Design review of the part built by this model. Coordinates are the model's own, in mm. Face numbers are marked on the shaded views. A direction names the side the tool comes from. Coordinates: 2 decimals unless noted, no trailing zeros. Write each loop counter-clockwise with the first axis right and the second up, starting at its lowest first coordinate (ties: lowest second). Pieces come first, ordered by that corner, then holes. Notation, with made-up numbers: (83.5, -23.75) -> (89.5, -23.75) arc R19 ccw to (89.5, -17.75) -> close; hole circle Ø2 at (55, 79.25). An arc over 180 degrees is marked (long way). Return JSON: item names as keys, results as strings. Group by question number.
from build123d import *

# Parameters (mm, degrees)
SALIENTE_EXTRUIR1_DEPTH      = 30
CORTAR_EXTRUIR1_DEPTH        = 5
CROQUIS3_W                   = 30
CROQUIS3_H                   = 25
CORTAR_EXTRUIR2_DEPTH        = 2
CROQUIS4_R                   = 1.35
CROQUIS4_R_2                 = 2.5
CORTAR_EXTRUIR3_DEPTH        = 5
CROQUIS5_W                   = 25
CROQUIS5_H                   = 25
CORTAR_EXTRUIR4_DEPTH        = 2
REDONDEO2_R                  = 20
REDONDEO3_R                  = 8
REDONDEO4_R                  = 2
SALIENTE_EXTRUIR2_DEPTH      = 9
SALIENTE_EXTRUIR2_DEPTH_BACK = 1
CORTAR_EXTRUIR5_START        = 9
CROQUIS10_W                  = 26
CROQUIS10_H                  = 14.6
CORTAR_EXTRUIR5_DEPTH        = 5
SALIENTE_EXTRUIR3_START      = 4
CROQUIS12_R                  = 3.6
CROQUIS12_R_2                = 2.1
SALIENTE_EXTRUIR3_DEPTH      = 3
CORTAR_EXTRUIR7_START        = -2
CROQUIS13_R                  = 2.1
CORTAR_EXTRUIR7_DEPTH        = 5
CORTAR_EXTRUIR8_START        = 9
CROQUIS14_W                  = 26
CROQUIS14_H                  = 5.4
CORTAR_EXTRUIR8_DEPTH        = 3.5
REDONDEO5_R                  = 3
SALIENTE_EXTRUIR4_DEPTH      = 1.5
SALIENTE_EXTRUIR4_DEPTH_BACK = 1.5
SALIENTE_EXTRUIR4_START      = -15


with BuildPart() as part:
    # Croquis1 → Saliente-Extruir1 (new body)
    with BuildSketch(Plane.XY):
        with BuildLine():
            Line((7, 0), (7, 5))
            Line((7, 5), (-33, 5))
            ThreePointArc((-33, 5), (-56.296113, -10.563595), (-70, -35))
            Line((-70, -35), (-70, -80))
            Line((-70, -80), (-65, -80))
            Line((-65, -80), (-65, -34.805195))
            ThreePointArc((-65, -34.805195), (-52.819114, -13.779819), (-32.805195, 0))
            Line((-32.805195, 0), (7, 0))
        make_face()
    extrude(amount=SALIENTE_EXTRUIR1_DEPTH)

    # Croquis2 → Cortar-Extruir1 (cut)
    with BuildSketch(Plane(origin=(0, 5, 0), x_dir=(1, 0, 0), z_dir=(0, 1, 0))):
        with BuildLine():
            Line((-11.4, -6.58), (-1.4, -6.58))
            ThreePointArc((-1.4, -6.58), (-0.05, -7.93), (-1.4, -9.28))
            Line((-1.4, -9.28), (-21.400001, -9.28))
            ThreePointArc((-21.400001, -9.28), (-22.75, -7.93), (-21.4, -6.58))
            Line((-21.4, -6.58), (-11.4, -6.58))
        make_face()
        with BuildLine():
            Line((-1.4, -20.72), (-21.400001, -20.72))
            ThreePointArc((-21.400001, -20.72), (-22.75, -22.07), (-21.4, -23.42))
            Line((-21.4, -23.42), (-11.4, -23.42))
            Line((-11.4, -23.42), (-1.4, -23.42))
            ThreePointArc((-1.4, -23.42), (-0.05, -22.07), (-1.4, -20.72))
        make_face()
    extrude(amount=-CORTAR_EXTRUIR1_DEPTH, mode=Mode.SUBTRACT)

    # Croquis3 → Cortar-Extruir2 (cut)
    with BuildSketch(Plane.XZ):
        with Locations((-11.4, 15)):
            Rectangle(CROQUIS3_W, CROQUIS3_H)
    extrude(amount=-CORTAR_EXTRUIR2_DEPTH, mode=Mode.SUBTRACT)

    # Croquis4 → Cortar-Extruir3 (cut)
    with BuildSketch(Plane.ZY.offset(70)):
        with Locations((22.071068, -54.528932)):
            Circle(CROQUIS4_R)
        with Locations((22.071068, -68.671068)):
            Circle(CROQUIS4_R)
        with Locations((7.928932, -68.671068)):
            Circle(CROQUIS4_R)
        with Locations((7.928932, -54.528932)):
            Circle(CROQUIS4_R)
        with Locations((15, -61.6)):
            Circle(CROQUIS4_R_2)
    extrude(amount=-CORTAR_EXTRUIR3_DEPTH, mode=Mode.SUBTRACT)

    # Croquis5 → Cortar-Extruir4 (cut)
    with BuildSketch(Plane.ZY.offset(70)):
        with Locations((15, -61.6)):
            Rectangle(CROQUIS5_W, CROQUIS5_H)
    extrude(amount=-CORTAR_EXTRUIR4_DEPTH, mode=Mode.SUBTRACT)

    # Redondeo2
    redondeo2_edges = [part.edges().sort_by_distance(p)[0] for p in [
        (-32.805195, 0, 15),
        (-65, -34.805195, 15),
        (-70, -35, 15),
        (-33, 5, 15),
    ]]
    fillet(redondeo2_edges, radius=REDONDEO2_R)

    # Redondeo3
    redondeo3_edges = [part.edges().sort_by_distance(p)[0] for p in [
        (7, 2.5, 0),
        (7, 2.5, 30),
    ]]
    fillet(redondeo3_edges, radius=REDONDEO3_R)

    # Redondeo4
    redondeo4_edges = [part.edges().sort_by_distance(p)[0] for p in [
        (-69, -49.1, 27.5),
        (-69, -74.1, 27.5),
        (-69, -74.1, 2.5),
        (-69, -49.1, 2.5),
        (3.6, 1, 27.5),
        (3.6, 1, 2.5),
        (-26.4, 1, 2.5),
        (-26.4, 1, 27.5),
    ]]
    fillet(redondeo4_edges, radius=REDONDEO4_R)

    # Croquis8 → Saliente-Extruir2 (add, two sides: drawn at the far end of the back side and taken through both)
    with BuildSketch(Plane.ZY.offset(70).offset(-SALIENTE_EXTRUIR2_DEPTH_BACK)):
        with BuildLine():
            Line((2.5, -72.1), (0, -72.1))
            Line((0, -72.1), (0, -80))
            Line((0, -80), (30, -80))
            Line((30, -80), (30, -72.1))
            Line((30, -72.1), (27.5, -72.1))
            ThreePointArc((27.5, -72.1), (26.914214, -73.514214), (25.5, -74.1))
            Line((25.5, -74.1), (4.5, -74.1))
            ThreePointArc((4.5, -74.1), (3.085786, -73.514214), (2.5, -72.1))
        make_face()
        with BuildLine():
            Line((2.5, -51.1), (0, -51.1))
            Line((0, -51.1), (0, -34))
            Line((0, -34), (30, -34))
            Line((30, -34), (30, -51.1))
            Line((30, -51.1), (27.5, -51.1))
            ThreePointArc((27.5, -51.1), (26.914214, -49.685786), (25.5, -49.1))
            Line((25.5, -49.1), (4.5, -49.1))
            ThreePointArc((4.5, -49.1), (3.085786, -49.685786), (2.5, -51.1))
        make_face()
    extrude(amount=SALIENTE_EXTRUIR2_DEPTH + SALIENTE_EXTRUIR2_DEPTH_BACK)

    # Croquis10 → Cortar-Extruir5 (cut)
    with BuildSketch(Plane.ZY.offset(70).offset(CORTAR_EXTRUIR5_START)):
        with Locations((15, -43.8)):
            Rectangle(CROQUIS10_W, CROQUIS10_H)
    extrude(amount=-CORTAR_EXTRUIR5_DEPTH, mode=Mode.SUBTRACT)

    # Croquis12 → Saliente-Extruir3 (add)
    with BuildSketch(Plane.ZY.offset(70).offset(SALIENTE_EXTRUIR3_START)):
        with Locations((5.5, -45.5)):
            Circle(CROQUIS12_R)
        with Locations(Location((5.5, -45.5, 0), (0, 0, 180))):
            Circle(CROQUIS12_R_2, mode=Mode.SUBTRACT)
    extrude(amount=SALIENTE_EXTRUIR3_DEPTH)

    # Croquis13 → Cortar-Extruir7 (cut)
    with BuildSketch(Plane.ZY.offset(74).offset(CORTAR_EXTRUIR7_START)):
        with Locations(Location((5.5, -45.5, 0), (0, 0, 180))):
            Circle(CROQUIS13_R)
    extrude(amount=CORTAR_EXTRUIR7_DEPTH, mode=Mode.SUBTRACT)

    # Croquis14 → Cortar-Extruir8 (cut)
    with BuildSketch(Plane.ZY.offset(70).offset(CORTAR_EXTRUIR8_START)):
        with Locations((15, -74.8)):
            Rectangle(CROQUIS14_W, CROQUIS14_H)
    extrude(amount=-CORTAR_EXTRUIR8_DEPTH, mode=Mode.SUBTRACT)

    # Redondeo5
    redondeo5_edges = [part.edges().sort_by_distance(p)[0] for p in [
        (-72, -80, 30),
        (-74.291633, -34, 30),
        (-74.291633, -34, 0),
        (-72, -80, 0),
    ]]
    fillet(redondeo5_edges, radius=REDONDEO5_R)

    # Croquis15 → Saliente-Extruir4 (add, two sides: drawn at the far end of the back side and taken through both)
    with BuildSketch(Plane.XY.offset(30).offset(SALIENTE_EXTRUIR4_START - SALIENTE_EXTRUIR4_DEPTH_BACK)):
        with BuildLine():
            Line((-65, -38.217888), (-28.4904, 0))
            ThreePointArc((-28.4904, 0), (-33.236938, -0.571403), (-37.712257, -2.252962))
            ThreePointArc((-37.712257, -2.252962), (-53.200641, -14.196528), (-63.566437, -30.782337))
            ThreePointArc((-63.566437, -30.782337), (-64.638339, -34.431646), (-65, -38.217888))
        make_face()
    extrude(amount=SALIENTE_EXTRUIR4_DEPTH + SALIENTE_EXTRUIR4_DEPTH_BACK)


solid = part.part
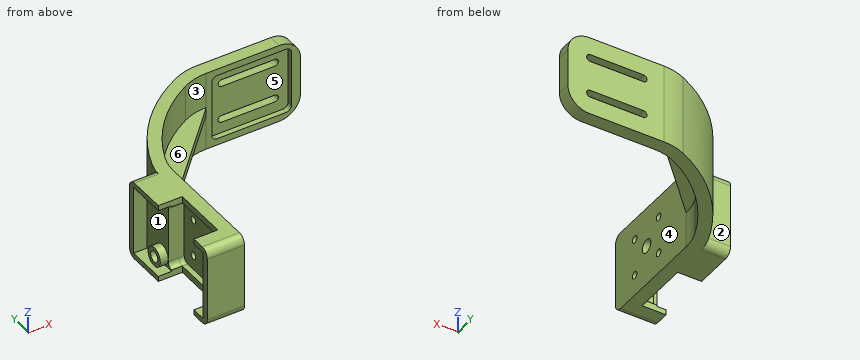
Q1. We need section B-B on y = -61.6. Write out the cut boundary in (x, z), plus the area to 3 significant figures.
Q2. For the marked faces 1, 2 and 3, list the 3-axis set-ups (+Z, -Z, +X, -X, +Y, -Y) from which the entire face can be reached by the end or side of a thin tool; tool diameter is ignored.
Q3. Wall thickness on L1, parallel to Y at x = -73.7, z = 5.5; L2, parallel to Y at x = -74.5, z = 3; L3, parallel to X at y = -73.5, z = 27.5: over which ranges is each line inside the solid? List them lowest first.
Q4. We need section D-D on y = -11. Write out the cut boundary in (x, z).
Q5. The part is to be moulded in two halves that separate along Z. For the marked faces 4, 5 and 6, say which applies: +Z half, -Z half, draft (parallel to the pull), parting line (faces both ways), or undercut.
Q6. For P1, Ø10, axis at x = -62.5, z = 5, coming from the +Y side; P2, Ø2, axis at x = -49, z = 17, coming from the -Y side; P3, Ø2, axis at y = -45, z = 6, coming from the -X side, all flat-tipped, find the tip position at first contact; note any pin that passes through.
Q7. We need section A-A on x = -71. Write out the cut boundary in (y, z), plus the area to 3 significant figures.
Q8. We need section C-C on z = 18.5. Write out the cut boundary in (x, y).
Findings below:
{
 "1": {"outline": "(-70, 0) -> (-65, 0) -> (-65, 12.5) -> (-68, 12.5) -> (-68, 2.5) -> (-70, 2.5) -> close; (-70, 27.5) -> (-68, 27.5) -> (-68, 17.5) -> (-65, 17.5) -> (-65, 30) -> (-70, 30) -> close", "area": "85.0 mm^2"},
 "2": {"face 1": "-X", "face 2": "+Z, -Z, -X, +Y", "face 3": "+Z, +X, -Y"},
 "3": {"L1": "y = -80 to -74.1, -49.1 to -47.6, -43.4 to -34", "L2": "y = -80 to -73.42, -48.09 to -42.91, -36.5 to -34", "L3": "x = -75.5 to -65"},
 "4": {"outline": "(-56.7, 0) -> (-50.06, 0) -> (-50.06, 13.5) -> (-39, 13.5) -> (-39, 16.5) -> (-50.06, 16.5) -> (-50.06, 30) -> (-56.7, 30) -> close"},
 "5": {"face 4": "draft", "face 5": "undercut", "face 6": "+Z half"},
 "6": {"P1": "stops at y = -11.9", "P2": "stops at y = -22.38", "P3": "stops at x = -72"},
 "7": {"outline": "(-80, 3) arc R3 ccw to (-77, 0) -> (-72.1, 0) -> (-72.1, 2.5) arc R2 cw to (-74.1, 4.5) -> (-74.1, 25.5) arc R2 cw to (-72.1, 27.5) -> (-72.1, 30) -> (-77, 30) arc R3 ccw to (-80, 27) -> close; (-51.1, 0) -> (-37, 0) arc R3 ccw to (-34, 3) -> (-34, 27) arc R3 ccw to (-37, 30) -> (-51.1, 30) -> (-51.1, 27.5) arc R2 cw to (-49.1, 25.5) -> (-49.1, 4.5) arc R2 cw to (-51.1, 2.5) -> close", "area": "646 mm^2"},
 "8": {"outline": "(-79, -80) -> (-65, -80) -> (-65, -38.22) arc R20 cw to (-63.57, -30.78) arc R55.34 cw to (-37.71, -2.25) arc R20 cw to (-28.49, 0) -> (-26.4, 0) -> (-26.4, 2) -> (3.6, 2) -> (3.6, 0) -> (7, 0) -> (7, 5) -> (-29.05, 5) arc R20 ccw to (-37.46, 3.14) arc R60.07 ccw to (-68.87, -31.43) arc R20 ccw to (-69.58, -34) -> (-79, -34) -> (-79, -36.5) -> (-74, -36.5) -> (-74, -49.1) -> (-68, -49.1) -> (-68, -74.1) -> (-75.5, -74.1) -> (-75.5, -77.5) -> (-79, -77.5) -> close"}
}
